Geometry check sheet. Reference: the model listing, model coordinates, mm. Face numbers are marked on the shaded views. Round coordinates to 2 decimals unless told otherwise and drop trailing zeros. Loops run counter-clockwise (first coordinate to the right, second up) from the corner with the lowest first, then second, coordinate; pieces in that order, holes last. Notation, with made-up numbers: (31, 47) - (65, 47) arc R34 ccw to (65, 84) - close; hole circle Ø8 at (27.5, 51). An arc over 180 degrees is marked (long way). Answer as CSV lines item,"result". Start each with the question number.
1) Cross-section at D-D on z = 19.5. Record the boundary of the cut face in (x, y).
2) Thickness scan on line 1 along Y through (x, z) = (4, -21); line 2 along X through (y, z) = (4.5, -8.5); line 3 along X through (y, z) = (2.95, -4). Record the ranges inside material, lowest first.
3) Cross-section at C-C on y = 0.95. Record the boundary of the cut face in (x, z), and give its area (3 significant figures).
4) Cross-section at B-B on x = -15. Record the boundary of the cut face in (y, z).
5) Depth check by flat-ended pin: P1, Ø3, axis at y = 4.5, z = 12, coming from the +X side. Enter the tip coordinate at first touch or a pass-through.
6) Draft check along Z on the marked faces 1 and 2. Enter one of: released by +Z, released by -Z, zero draft, split by the parting line, or undercut.
7) Cross-section at A-A on z = -6. Record the boundary of the cut face in (x, y).
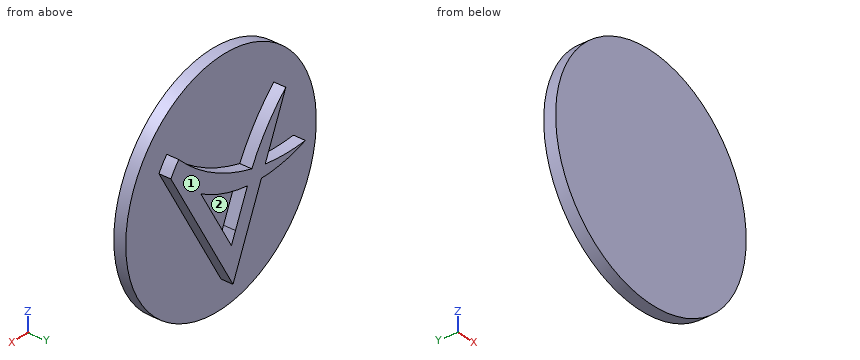
from build123d import *

# Parameters (mm, degrees)
SKETCH1_R           = 24.3
BOSS_EXTRUDE1_DEPTH = 2.5
BOSS_EXTRUDE3_DEPTH = 2.5


with BuildPart() as part:
    # Sketch1 → Boss-Extrude1 (new body)
    with BuildSketch(Plane(origin=(0, 0, 0), x_dir=(1, 0, 0), z_dir=(0, 1, 0))):
        Circle(SKETCH1_R)
    extrude(amount=BOSS_EXTRUDE1_DEPTH)

    # Sketch2 → Boss-Extrude3 (add)
    with BuildSketch(Plane(origin=(0, 2.5, 0), x_dir=(1, 0, 0), z_dir=(0, 1, 0))):
        with BuildLine():
            Line((-8.217088494, -0.523578651), (-13.461313625, -12.64466032))
            add(Edge.make_bspline(
                [(-13.461313625, -12.64466032), (-8.027902846, -7.603076106), (-4.786374516, -1.291203376)],
                knots=[0, 0, 0, 0.698779306, 0.698779306, 0.698779306], degree=2))
            ThreePointArc((-4.786374516, -1.291203376), (5.263745038, -5.505270352), (13.84122859, -12.227624065))
            ThreePointArc((13.84122859, -12.227624065), (14.904706404, -10.90615084), (15.842456672, -9.492679587))
            Line((15.842456672, -9.492679587), (0, 18.468741136))
            Line((0, 18.468741136), (-7.240743071, 1.733067912))
            ThreePointArc((-7.240743071, 1.733067912), (-12.934133358, 1.380884752), (-18.468741136, 0))
            ThreePointArc((-18.468741136, 0), (-13.32639579, 0.061652646), (-8.217088494, -0.523578651))
        make_face()
        with BuildLine():
            ThreePointArc((8.198670855, -2.878510194), (2.478425995, -0.121109089), (-3.681028203, 1.423425177))
            Line((-3.681028203, 1.423425177), (-0.630983691, 8.473053617))
            Line((-0.630983691, 8.473053617), (0.407335967, 10.872942458))
            Line((0.407335967, 10.872942458), (2.461520314, 7.247373901))
            Line((2.461520314, 7.247373901), (8.198670855, -2.878510194))
        make_face(mode=Mode.SUBTRACT)
    extrude(amount=BOSS_EXTRUDE3_DEPTH)


solid = part.part
Answer block:
1,outline,"(-14.5, 0) - (14.5, 0) - (14.5, 2.5) - (-14.5, 2.5) - close"
2,line 1,"y = 0 to 2.5"
2,line 2,"x = -4.31 to -0.62, 1.75 to 5.65"
2,line 3,"x = -6.26 to -2.57, 4.3 to 8.2"
3,outline,"circle Ø48.6 at (0, 0)"
3,area,"1,860 mm^2"
4,outline,"(0, -19.12) - (2.5, -19.12) - (2.5, -0.99) - (5, -0.99) - (5, -0.11) - (2.5, -0.11) - (2.5, 19.12) - (0, 19.12) - close"
5,P1,"stops at x = 15.19"
6,face 1,"zero draft"
6,face 2,"undercut"
7,outline,"(-23.55, 0) - (23.55, 0) - (23.55, 2.5) - (7.06, 2.5) - (7.06, 5) - (3.17, 5) - (3.17, 2.5) - (-1.7, 2.5) - (-1.7, 5) - (-5.39, 5) - (-5.39, 2.5) - (-23.55, 2.5) - close"
